Verification items for the finished model (mm, model axes). A direction names the side the tool comes from. Coordinates: 2 decimals unless noted, no trailing zeros. Write each loop counter-clockwise with the first axis right and the second up, starting at its lowest first coordinate (ties: lowest second). Pieces come first, ordered by that corner, then holes. Notation, with made-up numbers: M 32.25,-9 L 88.25,-9 A13 ccw 88.25,6 Z; hole C -39,88 d1. An arc over 180 degrees is marked long. Answer in a Markdown table with one row per item.
from build123d import *

# Parameters (mm, degrees)
BOSS_EXTRUDE1_DEPTH = 4.5


with BuildPart() as part:
    # Sketch1 → Boss-Extrude1 (new body)
    with BuildSketch(Plane.XY):
        with BuildLine():
            Line((71.318213966, -108.561967819), (29.643230329, 10.3859037))
            ThreePointArc((29.643230329, 10.3859037), (-6.509198083, 30.728137599), (-31.308299059, -2.525571229))
            ThreePointArc((-31.308299059, -2.525571229), (-9.015287266, -74.800110093), (41.79304757, -130.827785878))
            ThreePointArc((41.79304757, -130.827785878), (64.686923189, -130.477223183), (71.318213966, -108.561967819))
        make_face()
        with BuildLine():
            Line((66.599457149, -110.215247618), (24.924473511, 8.732623901))
            ThreePointArc((24.924473511, 8.732623901), (-5.473031562, 25.836679847), (-26.324488321, -2.123538241))
            ThreePointArc((-26.324488321, -2.123538241), (-4.670950627, -72.32488502), (44.679949278, -126.7454093))
            ThreePointArc((44.679949278, -126.7454093), (61.676381409, -126.485151265), (66.599457149, -110.215247618))
        make_face(mode=Mode.SUBTRACT)
    extrude(amount=BOSS_EXTRUDE1_DEPTH)


solid = part.part
1) Sectioned sample at A-A (z = 3.05). Record the cut outline in (x, y), then the cut area to 3 significant figures.
Response values:
| item | result |
|---|---|
| outline | M -31.31,-2.53 A174.31 ccw 41.79,-130.83 A19.41 ccw 71.32,-108.56 L 29.64,10.39 A31.41 ccw Z; hole M -26.32,-2.12 A169.31 ccw 44.68,-126.75 A14.41 ccw 66.6,-110.22 L 24.92,8.73 A26.41 ccw Z |
| area | 2,010 mm² |
2) Release check for a two-part mould opening along Y. For faces 1 (the face through (50.772, -49.921, 2.218)), 2 (the face through (43, -39, 4.5)), 3 (the face through (-5.181, -71.423, 2.218)) record: +Y half, -Y half, draft (parallel to the pull), parting line (faces both ways), or undercut.
Response values:
| item | result |
|---|---|
| face 1 | +Y half |
| face 2 | draft |
| face 3 | undercut |
3) Tool access check on faces 4 (the face through (43, -39, 0)), 5 (the face through (-4.95, 25.94, 2.22)). Record the directions out of +Z, -Z, +X, -X, +Y, -Y that give a thin tool (end or side, any length) a straight path to the whole face; none if there is none.
Response values:
| item | result |
|---|---|
| face 4 | -Z, +X, -X, +Y, -Y |
| face 5 | +Z, -Z |
4) Thickness scan on L1, parallel to X at y = -115, z = 1.5; L2, parallel to X at y = 17.5, z = 4.05; L3, parallel to Y at x = 3.5, z = 3.9. Record the ranges inside material, lowest first. Write a range as [from, to].
Response values:
| item | result |
|---|---|
| L1 | x = [22.5, 29.89], [67.41, 72.41] |
| L2 | x = [-26.08, -19.78], [19.78, 26.08] |
| L3 | y = [-93.77, -85.27], [26.18, 31.21] |
5) Depth check by flat-ended pin: pin 1 (12 mm diameter, centred on x = 32.5, y = 8, fed in from +Z); pin 2 (1.5 mm diameter, centred on y = -86.5, z = 1.5, fed in from +X); pin 3 (1.5 mm diameter, centred on x = 58.5, z = 1.5, fed in from -Y). Enter the tip coordinate at first touch or a pass-through.
Response values:
| item | result |
|---|---|
| pin 1 | stops at z = 4.5 |
| pin 2 | stops at x = 63.85 |
| pin 3 | stops at y = -133.8 |
6) Sectioned sample at C-C (x = 63). Record the cut outline in (y, z), then the cut area to 3 significant figures.
Response values:
| item | result |
|---|---|
| outline | M -131.62,0 L -125.36,0 L -125.36,4.5 L -131.62,4.5 Z; M -99.94,0 L -84.82,0 L -84.82,4.5 L -99.94,4.5 Z |
| area | 96.2 mm² |
7) Sectioned sample at B-B (y = 18). Record the cut outline in (x, z), then the cut area to 3 significant figures.
Response values:
| item | result |
|---|---|
| outline | M -25.74,0 L -19.33,0 L -19.33,4.5 L -25.74,4.5 Z; M 19.33,0 L 25.74,0 L 25.74,4.5 L 19.33,4.5 Z |
| area | 57.7 mm² |
